Autodesk Inventor part; units mm, degrees
ref_plane "YZ Plane" through (0, 0, 0) normal (1, 0, 0) x (0, 1, 0)
ref_plane "XZ Plane" through (0, 0, 0) normal (0, 1, 0) x (-1, 0, 0)
ref_plane "XY Plane" through (0, 0, 0) normal (0, 0, 1) x (1, 0, 0)
sketch "Эскиз1" plane through (0, 0, 0) normal (0, 0, 1) x (1, 0, 0)
  line L0 (0, 0) -> (44.5, 0)
  line L1 (44.5, 0) -> (44.5, 35.5)
  line L2 (44.5, 35.5) -> (0, 35.5)
  line L3 (0, 35.5) -> (0, 0)
  dimension "d0" = 44.5
  dimension "d1" = 35.5
extrude "Выдавливание1" add sketch "Эскиз1" along normal blind 1.7
sketch "Эскиз2" plane through (0, 0, 1.7) normal (0, 0, 1) x (1, 0, 0)
  line L0 (0, 0) -> (44.5, 0)
  line L1 (44.5, 0) -> (44.5, 3.5)
  line L2 (44.5, 0) -> (44.5, 35.5)
  line L3 (44.5, 3.5) -> (41, 3.5)
  line L4 (44.5, 35.5) -> (44.5, 32)
  line L5 (44.5, 32) -> (41, 32)
  dimension "d4" = 3.5
  dimension "d5" = 3.5
  dimension "d6" = 3.5
  dimension "d7" = 3.5
hole "Отверстие1" at (41, 32, 1.7) at (41, 3.5, 1.7) direction (0, 0, -1) diameter 3.35 depth 15
sketch "Эскиз3" plane through (0, 0, 0) normal (0, 0, -1) x (-1, 0, 0)
  line L0 (-44.5, 0) -> (-44.5, 35.5)
  line L1 (-44.5, 0) -> (-44.5, 9.25)
  line L2 (-44.5, 9.25) -> (-27.5, 9.25)
  line L3 (-27.5, 9.25) -> (-27.5, 26.25)
  line L4 (-27.5, 26.25) -> (-44.5, 26.25)
  line L5 (-44.5, 26.25) -> (-44.5, 9.25)
  line L6 (-36, 26.25) -> (-36, 27.75)
  line L7 (-36, 9.25) -> (-36, 7.75)
  circle A0 centre (-36, 7.75) radius 2.5
  circle A1 centre (-36, 27.75) radius 2.5
  line L8 (-38.5, 27.75) -> (-33.5, 27.75)
  line L9 (-33.5, 27.75) -> (-33.5, 26.25)
  line L10 (-33.5, 26.25) -> (-38.5, 26.25)
  line L11 (-38.5, 26.25) -> (-38.5, 27.75)
  line L12 (-33.5, 7.75) -> (-38.5, 7.75)
  line L13 (-38.5, 7.75) -> (-38.5, 9.25)
  line L14 (-38.5, 9.25) -> (-33.5, 9.25)
  line L15 (-33.5, 9.25) -> (-33.5, 7.75)
  point P0 (0, 0)
  dimension "d20" = 5
  dimension "d21" = 5
  dimension "d15" = 9.25
  dimension "d16" = 17
  dimension "d17" = 17
  dimension "d18" = 1.5
  dimension "d19" = 1.5
extrude "Выдавливание2" add sketch "Эскиз3" along normal blind 8
sketch "Эскиз4" plane through (0, 0, -8) normal (0, 0, -1) x (-1, 0, 0)
  line L0 (-44.5, 0) -> (-44.5, 35.5)
  line L1 (-44.5, 17.75) -> (-27.5, 17.75)
  line L2 (-27.5, 26.25) -> (-27.5, 9.25)
  circle A0 centre (-36, 17.75) radius 8.5
  point P0 (0, 0)
extrude "Выдавливание3" add sketch "Эскиз4" along normal blind 14
equation "\"d4\" = d6"
equation "\"d5\" = d6"
equation "\"d7\" = d6"
properties part number "Техническое зрение OpenMV"
Here's how the part is built. I have some questions about the finished solid (model axes, mm). A direction names the side the tool comes from. Coordinates: 2 decimals unless noted, no trailing zeros. Write each loop counter-clockwise with the first axis right and the second up, starting at its lowest first coordinate (ties: lowest second). Pieces come first, ordered by that corner, then holes. Notation, with made-up numbers: (-1.5, 7) -> (48.5, 7) arc R24 cw to (48.5, 41) -> close; hole circle Ø10 at (73, 68). An arc over 180 degrees is marked (long way). Use a Markdown table: item, result. Add a question column.
(1) I'm going to push flat-ended pins straight in: P1, Ø2, axis at x = 29, z = -19, coming from the -Y side; P2, Ø1.6, axis at y = 8, z = -2.5, coming from the -X side; P3, Ø3, axis at x = 29.5, z = -6, coming from the +Y side. Where does each tip first touch, or does it pass through?
(2) Please list where these lines run through material, in increasing order: line 1 (Y direction, x = 41, z = 1) (3 decimals); line 2 (X direction, y = 32, z = 0.55) (3 decimals); line 3 (Z direction, x = 28, y = 32).
(3) For faces 4 (the flat face through (38.5, 8, -4)), 5 (the flat face through (41, 26.25, -4)), 6 (the cylindrical face through (36.05, 30.25, -3.94)), 7 (the flat face through (33.5, 9, -4)), 8 (the cylindrical face through (37.84, 26.05, -14.9)), which set-ups out of +Z, -Z, +X, -X, +Y, -Y let a thin tool reach every point of the face, with its end or its side?
(4) We'd pull the mould along Y, two halves only. Please class faces 1 (the flat face through (27.5, 18, -4)), 2 (the cylindrical face through (39.34, 3.72, 0.84)), 3 (the flat face through (22, 0, 1)): +Y half, -Y half, draft (parallel to the pull), parting line (faces both ways), or undercut.
(5) If we section it at D-D, the plane x = 36: Write out the boundary of the cut face in (y, z), and give its area (3 significant figures).
(6) If we section it at A-A, the plane y = 32: Write out the boundary of the cut face in (x, z) (3 decimals).
(7) If we section it at C-C, the plane y = 27: Write out the boundary of the cut face in (x, z), and give its area (3 significant figures).
(8) If we section it at B-B, the plane z = -3: Write out the boundary of the cut face in (x, y), and give its area (3 significant figures).
Outcome:
| question | item | result |
|---|---|---|
| 1 | P1 | stops at y = 11.73 |
| 1 | P2 | stops at x = 33.5 |
| 1 | P3 | stops at y = 26.25 |
| 2 | line 1 | y = 0 to 1.825, 5.175 to 30.325, 33.675 to 35.5 |
| 2 | line 2 | x = 0 to 39.325, 42.675 to 44.5 |
| 2 | line 3 | z = 0 to 1.7 |
| 3 | face 4 | -Z, +X, -Y |
| 3 | face 5 | -Z, +X, +Y |
| 3 | face 6 | -Z, +Y |
| 3 | face 7 | -Z, -X, -Y |
| 3 | face 8 | -Z |
| 4 | face 1 | draft |
| 4 | face 2 | undercut |
| 4 | face 3 | -Y half |
| 5 | outline | (0, 0) -> (5.25, 0) -> (5.25, -8) -> (9.25, -8) -> (9.25, -22) -> (26.25, -22) -> (26.25, -8) -> (30.25, -8) -> (30.25, 0) -> (35.5, 0) -> (35.5, 1.7) -> (0, 1.7) -> close |
| 5 | area | 498 mm^2 |
| 6 | outline | (0, 0) -> (39.325, 0) -> (39.325, 1.7) -> (0, 1.7) -> close; (42.675, 0) -> (44.5, 0) -> (44.5, 1.7) -> (42.675, 1.7) -> close |
| 7 | outline | (0, 0) -> (33.5, 0) -> (33.5, -8) -> (38.5, -8) -> (38.5, 0) -> (44.5, 0) -> (44.5, 1.7) -> (0, 1.7) -> close |
| 7 | area | 116 mm^2 |
| 8 | outline | (27.5, 9.25) -> (33.5, 9.25) -> (33.5, 7.75) arc R2.5 ccw to (38.5, 7.75) -> (38.5, 9.25) -> (44.5, 9.25) -> (44.5, 26.25) -> (38.5, 26.25) -> (38.5, 27.75) arc R2.5 ccw to (33.5, 27.75) -> (33.5, 26.25) -> (27.5, 26.25) -> close |
| 8 | area | 324 mm^2 |
